```python
from build123d import *

# Parameters (mm, degrees)
SKETCH_1_W          = 40
SKETCH_1_H          = 1
EXTRUDE_1_DEPTH     = 66
SKETCH_2_W          = 24
SKETCH_2_H          = 35
EXTRUDE_2_DEPTH     = 8.5
SKETCH_3_R          = 1.5
CUT_EXTRUDE_1_DEPTH = 78.757636281


with BuildPart() as part:
    # ｽｹｯﾁ1 → ﾎﾞｽ - 押し出し1 (new body)
    with BuildSketch(Plane.XY):
        with Locations((20, 0.5)):
            Rectangle(SKETCH_1_W, SKETCH_1_H)
    extrude(amount=EXTRUDE_1_DEPTH)

    # ｽｹｯﾁ2 → ﾎﾞｽ - 押し出し2 (add)
    with BuildSketch(Plane.XZ):
        with Locations((20, 33)):
            Rectangle(SKETCH_2_W, SKETCH_2_H)
    extrude(amount=EXTRUDE_2_DEPTH)

    # ｽｹｯﾁ3 → ｶｯﾄ - 押し出し1 (cut, through all)
    with BuildSketch(Plane(origin=(0, 1, 0), x_dir=(1, 0, 0), z_dir=(0, 1, 0))):
        with Locations(Location((3, -13, 0), (0, 0, 180))):
            Circle(SKETCH_3_R)
        with Locations(Location((37, -13, 0), (0, 0, 180))):
            Circle(SKETCH_3_R)
        with Locations(Location((3, -53, 0), (0, 0, 180))):
            Circle(SKETCH_3_R)
        with Locations(Location((37, -53, 0), (0, 0, 180))):
            Circle(SKETCH_3_R)
    extrude(amount=-CUT_EXTRUDE_1_DEPTH, mode=Mode.SUBTRACT)


solid = part.part
```
Read the model definition and answer for the solid it produces. Units are mm, in the model's axes. A direction names the side the tool comes from. Round coordinates to 2 decimals unless told otherwise and drop trailing zeros. Write each loop counter-clockwise with the first axis right and the second up, starting at its lowest first coordinate (ties: lowest second). Pieces come first, ordered by that corner, then holes. Notation, with made-up numbers: (62, 49.5) - (81, 49.5) arc R23 cw to (81, 85.5) - close; hole circle Ø5 at (2.5, -32.75). An arc over 180 degrees is marked (long way). Use CSV: the item, a comma, the result in double quotes.
Q1. Find section D-D, the plane z = 22. Write down the section's boundary in (x, y), then the cut area to 3 significant figures.
Values:
outline,"(0, 0) - (8, 0) - (8, -8.5) - (32, -8.5) - (32, 0) - (40, 0) - (40, 1) - (0, 1) - close"
area,"244 mm²"
Q2. Find section C-C, the plane x = 16.5. Write down the section's boundary in (y, z).
Values:
outline,"(-8.5, 15.5) - (0, 15.5) - (0, 0) - (1, 0) - (1, 66) - (0, 66) - (0, 50.5) - (-8.5, 50.5) - close"
Q3. Each of these flat-tipped pins is pushed along its axis until it touches: pin 1 Ø4 at (y, z) = (-2.5, 36) entering from +X; pin 2 Ø2.5 at (x, y) = (17.5, -2.5) entering from +Z; pin 3 Ø5 at (x, y) = (15, -4.5) entering from -Z; pin 4 Ø3.5 at (x, z) = (3, 13) entering from +Y. Where does it stop, or does it pass through?
Values:
pin 1,"stops at x = 32"
pin 2,"stops at z = 50.5"
pin 3,"stops at z = 15.5"
pin 4,"stops at y = 1"
Q4. Straight lines are drawn through the part: line 1 along Z through (x, y) = (37, 0.35); line 2 along X through (y, z) = (-5.25, 38.5); line 3 along Z through (x, y) = (11, -6.5). For each, find the intervals that lie inside material, in ascending order.
Values:
line 1,"z = 0 to 11.5, 14.5 to 51.5, 54.5 to 66"
line 2,"x = 8 to 32"
line 3,"z = 15.5 to 50.5"
Q5. Find section A-A, the plane z = 13. Write down the section's boundary in (x, y), then the cut area to 3 significant figures.
Values:
outline,"(0, 0) - (1.5, 0) - (1.5, 1) - (0, 1) - close; (4.5, 0) - (35.5, 0) - (35.5, 1) - (4.5, 1) - close; (38.5, 0) - (40, 0) - (40, 1) - (38.5, 1) - close"
area,"34.0 mm²"
Q6. A tool of negligible diameter and unlimited length cuts with its end or side. For faces 1 (the flat face through (20, -4, 15.5)), 2 (the flat face through (32, -4, 33)), 3 (the cylindrical face through (38.2, 0.5, 12.1)), from which of +Z, -Z, +X, -X, +Y, -Y can it reach the whole face along a straight path? Write none if from no direction.
Values:
face 1,"-Z, +X, -X, -Y"
face 2,"+Z, -Z, +X, -Y"
face 3,"+Y, -Y"
Q7. Find section B-B, the plane x = 3. Write down the section's boundary in (y, z).
Values:
outline,"(0, 0) - (1, 0) - (1, 11.5) - (0, 11.5) - close; (0, 14.5) - (1, 14.5) - (1, 51.5) - (0, 51.5) - close; (0, 54.5) - (1, 54.5) - (1, 66) - (0, 66) - close"
Q8. Determine the mould class of faces 4 (the flat face through (8, -4, 33)), 5 (the flat face through (20, -4, 50.5)), 6 (the cylindrical face through (38.2, 0.5, 52.1)) for opening direction Z: +Z half, -Z half, draft (parallel to the pull), parting line (faces both ways), or undercut.
Values:
face 4,"draft"
face 5,"+Z half"
face 6,"undercut"
